Part model, mm, in its own coordinate system. Face numbers are marked on the shaded views. A direction names the side the tool comes from. Coordinates: 2 decimals unless noted, no trailing zeros. Write each loop counter-clockwise with the first axis right and the second up, starting at its lowest first coordinate (ties: lowest second). Pieces come first, ordered by that corner, then holes. Notation, with made-up numbers: (-7, -24) -> (29, -24) arc R16 ccw to (29, -17) -> close; hole circle Ø4 at (-24, 26). An arc over 180 degrees is marked (long way). Write item = value, one per line. Start each with the question number.
Q1. Band-saw the part on A-A, the plane z = 0. List the corners of the cut face in (x, y), plus the area to 3 significant figures.
Q2. Band-saw the part on B-B, the plane x = -2.25. List the corners of the cut face in (y, z), plus the area to 3 significant figures.
Q3. Band-saw the part on D-D, the plane y = 6.5. List the corners of the cut face in (x, z), plus the area to 3 significant figures.
Q4. Pull direction X, two halves, no side cores. Call the marked faces 4, 5, 6 and 7: released by +X, released by -X, zero draft, split by the parting line, or undercut.
Q5. Probe line 1 (X direction, y = 3.6, z = 0); line 2 (X direction, y = 4.35, z = 0); line 3 (Y direction, x = 2, z = 1.75). List the from-to ranges inside material, lowest first.
Q6. Tool access for the marked faces 1, 2 and 3: list every direction of +Z, -Z, +X, -X, +Y, -Y with a clear straight run to the whole face (end or side of a thin tool).
Q7. Pin check, flat tips, straight feed: P1, Ø1, axis at y = 1.5, z = -2.5, coming from the -X side; P2, Ø3, axis at y = 3, z = -0.5, coming from the -X side; P3, Ø2, axis at y = 11, z = -1.5, coming from the +X side; P4, Ø3, axis at x = -0.5, y = 12, coming from the +Z side. Stop position of each tip, or through.
Q8. Band-saw the part on C-C, the plane y = 3.25. List the corners of the cut face in (x, z), plus the area to 3 significant figures.
from build123d import *

# Parameters (mm, degrees)
SKETCH1_R           = 5
SKETCH1_R_2         = 3
BOSS_EXTRUDE1_DEPTH = 4
SKETCH2_R           = 5
BOSS_EXTRUDE2_DEPTH = 4
SKETCH3_R           = 2.5
BOSS_EXTRUDE3_DEPTH = 6
SKETCH4_R           = 3
CUT_EXTRUDE1_DEPTH  = 2
BOSS_EXTRUDE4_DEPTH = 6


with BuildPart() as part:
    # Sketch1 → Boss-Extrude1 (new body)
    with BuildSketch(Plane(origin=(0, 0, 0), x_dir=(1, 0, 0), z_dir=(0, 1, 0))):
        with Locations((-1, 0)):
            Circle(SKETCH1_R)
        Circle(SKETCH1_R_2, mode=Mode.SUBTRACT)
    extrude(amount=BOSS_EXTRUDE1_DEPTH)

    # Sketch2 → Boss-Extrude2 (add)
    with BuildSketch(Plane(origin=(0, 4, 0), x_dir=(1, 0, 0), z_dir=(0, 1, 0))):
        with Locations((1, 0)):
            Circle(SKETCH2_R)
    extrude(amount=BOSS_EXTRUDE2_DEPTH)

    # Sketch3 → Boss-Extrude3 (add)
    with BuildSketch(Plane(origin=(0, 8, 0), x_dir=(1, 0, 0), z_dir=(0, 1, 0))):
        Circle(SKETCH3_R)
    extrude(amount=BOSS_EXTRUDE3_DEPTH)

    # Sketch4 → Cut-Extrude1 (cut)
    with BuildSketch(Plane.XZ.offset(-4)):
        Circle(SKETCH4_R)
    extrude(amount=-CUT_EXTRUDE1_DEPTH, mode=Mode.SUBTRACT)

    # Sketch6 → Boss-Extrude4 (add, through all)
    with BuildSketch(Plane.XZ.offset(-6)):
        with BuildLine():
            ThreePointArc((3, 0), (2.711088342, 1.284523258), (1.9, 2.321637353))
            Line((1.9, 2.321637353), (1.9, -2.321637353))
            ThreePointArc((1.9, -2.321637353), (2.711088342, -1.284523258), (3, 0))
        make_face()
    extrude(amount=BOSS_EXTRUDE4_DEPTH)


solid = part.part
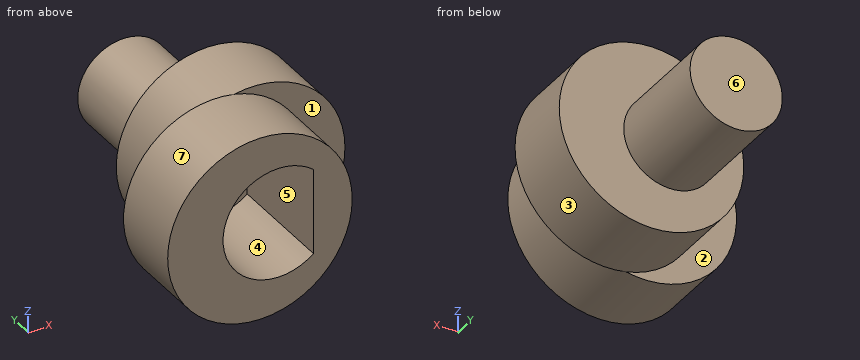
Ans:
q1.outline = (-6, 0) -> (-3, 0) -> (-3, 6) -> (1.9, 6) -> (1.9, 0) -> (4, 0) -> (4, 4) -> (6, 4) -> (6, 8) -> (2.5, 8) -> (2.5, 14) -> (-2.5, 14) -> (-2.5, 8) -> (-4, 8) -> (-4, 4) -> (-6, 4) -> close
q1.area = 80.6 mm2
q2.outline = (0, -4.84) -> (4, -4.84) -> (4, -3.8) -> (8, -3.8) -> (8, -1.09) -> (14, -1.09) -> (14, 1.09) -> (8, 1.09) -> (8, 3.8) -> (4, 3.8) -> (4, 4.84) -> (0, 4.84) -> (0, 1.98) -> (6, 1.98) -> (6, -1.98) -> (0, -1.98) -> close
q2.area = 58.4 mm2
q3.outline = circle Ø10 at (1, 0)
q3.area = 78.5 mm2
q4.face_4 = undercut
q4.face_5 = undercut
q4.face_6 = zero draft
q4.face_7 = split by the parting line
q5.line_1 = -6 to -3, 1.9 to 4
q5.line_2 = -4 to -3, 1.9 to 6
q5.line_3 = 0 to 8
q6.face_1 = +X, -Y
q6.face_2 = -X, +Y
q6.face_3 = +Y
q7.P1 = -5.58
q7.P2 = -6
q7.P3 = 2.45
q7.P4 = 2.5
q8.outline = circle Ø10 at (-1, 0); hole (1.9, -2.32) -> (1.9, 2.32) arc R3 ccw (long way) to start
q8.area = 53.8 mm2
